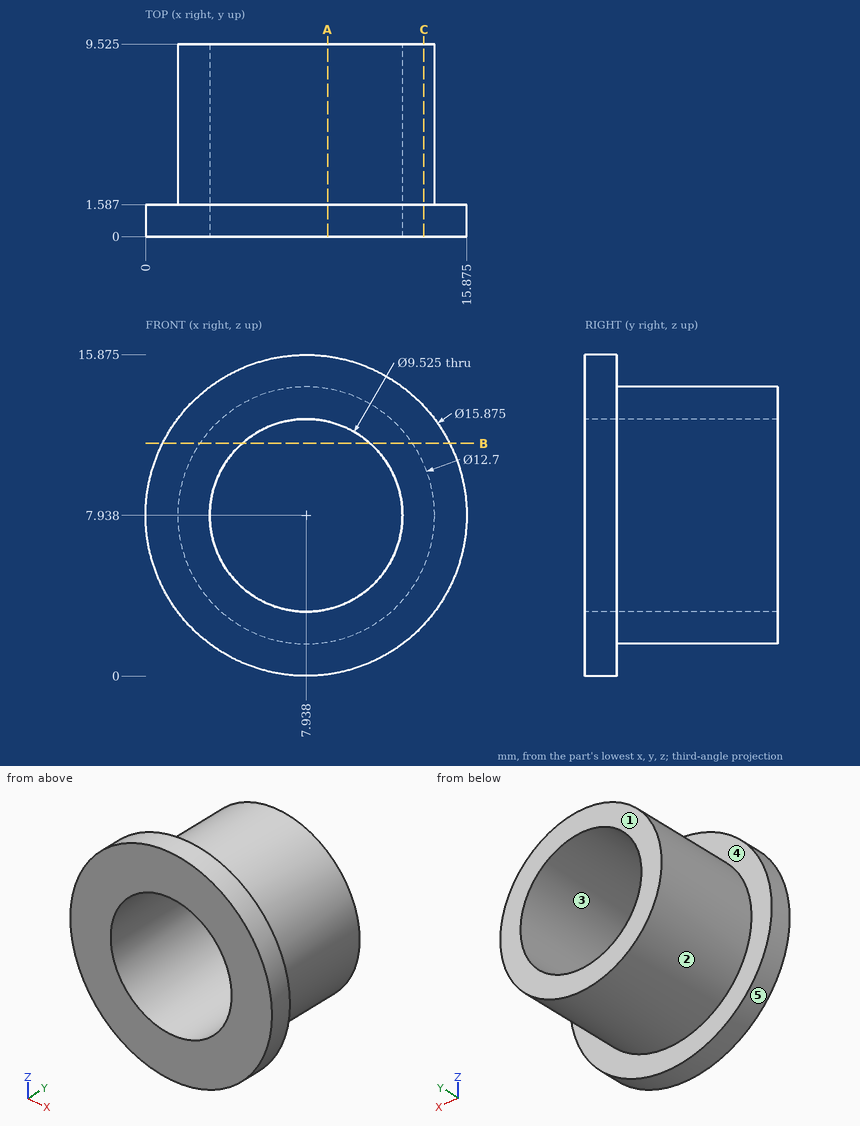
Answer from the drawing. Dimensions are ordinates in mm from the lowest x, y and z of the part. A direction names the side the tool comes from. Coordinates: 2 decimals unless noted, no trailing zeros. Write each loop counter-clockwise with the first axis right and the second up, starting at its lowest first coordinate (ties: lowest second). Pieces come first, ordered by that corner, then holes. Notation, with made-up numbers: (59.5, 57) - (70.5, 57) arc R19 ccw to (70.5, 89) - close; hole circle Ø1 at (64.25, -0.75). An arc over 180 degrees is marked (long way). Return JSON: item names as keys, results as strings.
1. The part is cut by section A-A on x = 9. Determine the outline of the cut face in (y, z) (1 decimal).
Final values:
{"outline": "(0, 0.1) - (1.6, 0.1) - (1.6, 1.7) - (9.5, 1.7) - (9.5, 3.3) - (0, 3.3) - close; (0, 12.6) - (9.5, 12.6) - (9.5, 14.2) - (1.6, 14.2) - (1.6, 15.8) - (0, 15.8) - close"}
2. The part is cut by section C-C on x = 13.75. Determine the outline of the cut face in (y, z) (1 decimal).
Final values:
{"outline": "(0, 2.5) - (1.6, 2.5) - (1.6, 5.4) - (9.5, 5.4) - (9.5, 10.5) - (1.6, 10.5) - (1.6, 13.3) - (0, 13.3) - close"}
3. For a pull along Z with two mould halves and no side action, classify the marked faces 3, 4 and 5 as +Z half, -Z half, draft (parallel to the pull), parting line (faces both ways), or undercut.
Final values:
{"face 3": "undercut", "face 4": "draft", "face 5": "parting line"}
4. Which of the six approach directions +Z, -Z, +X, -X, +Y, -Y give full straight-line access (tool end or side, diameter ignored) to the marked faces 1 and 2?
Final values:
{"face 1": "+Z, -Z, +X, -X, +Y", "face 2": "+Y"}
5. The part is cut by section B-B on z = 11.5. Determine the outline of the cut face in (x, y) (1 decimal).
Final values:
{"outline": "(0.8, 0) - (4.8, 0) - (4.8, 9.5) - (2.7, 9.5) - (2.7, 1.6) - (0.8, 1.6) - close; (11.1, 0) - (15, 0) - (15, 1.6) - (13.2, 1.6) - (13.2, 9.5) - (11.1, 9.5) - close"}
6. Each of these flat-tipped pins is pushed along its axis until it touches: pin 1 Ø2 at (y, z) = (4.5, 5.5) entering from -X; pin 2 Ø1 at (y, z) = (7, 11) entering from +X; pin 3 Ø3 at (y, z) = (5, 13) entering from -X. Where does it stop, or does it pass through?
Final values:
{"pin 1": "x = 1.75", "pin 2": "x = 13.75", "pin 3": "x = 2.68"}
7. Consider line 1 along Y through (x, z) = (0.5, 10.25); line 2 along X through (y, z) = (4, 8.25) (1 decimal); line 3 along X through (y, z) = (7.25, 9) (1 decimal). Determine where each line is inside the solid, lowest interval first.
Final values:
{"line 1": "0 to 1.59", "line 2": "1.6 to 3.2, 12.7 to 14.3", "line 3": "1.7 to 3.3, 12.6 to 14.2"}
